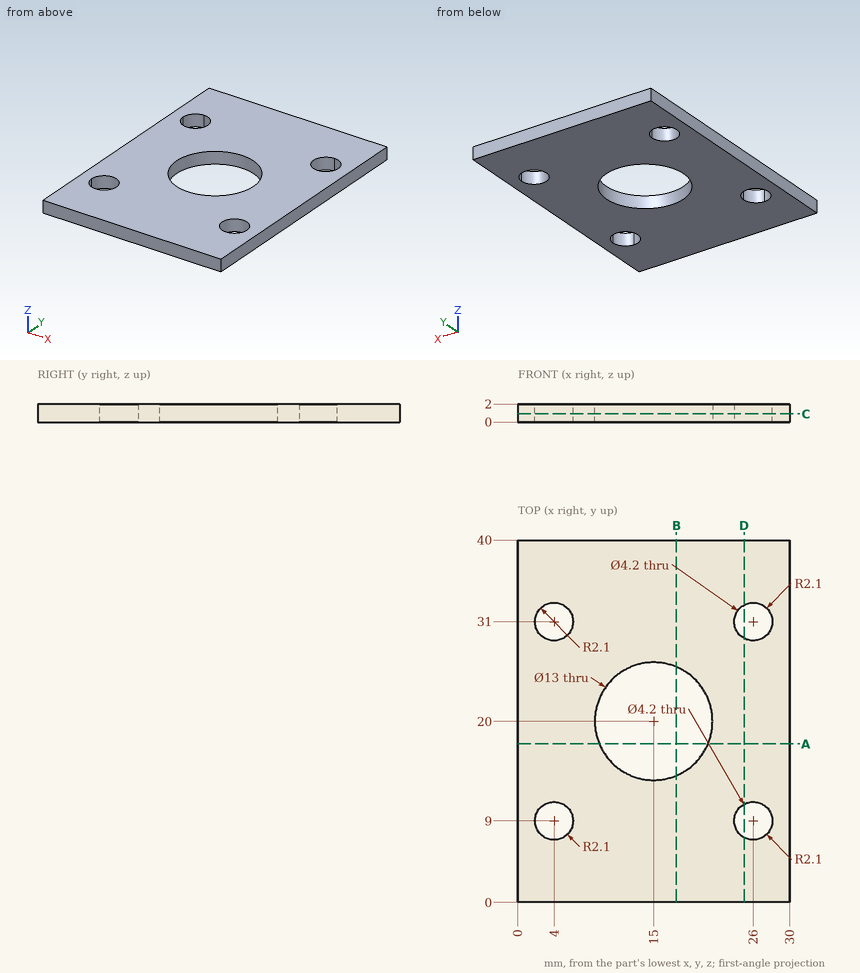
Geometry check sheet. Reference: drawing and pictorial views, mm from the part's lowest x, y, z. Give positions to 0.01 mm unless a question says otherwise; leave off trailing zeros. Order: outer loops, then holes, each group sorted by start corner. A loop starts at its lowest first (then second) coordinate and runs counter-clockwise, first axis right, second up. Notation, with made-up numbers: M 68,77 L 104,77 A21 ccw 104,110 Z; hole C -9.5,28 d4. An arc over 180 degrees is marked long. Answer in a Markdown table with one row per item. Add a question column.
Item 1: Gauge pin test, flat end, axial feed: pin 1 (2.5 mm diameter, centred on x = 26, y = 31, fed in from +Z). Record the tip position at first contact, or that the pin passes through.
Item 2: Scan lines: probe 1 along X at (y, z) = (9, 0.75); probe 2 along Y at (x, z) = (26, 0.1); probe 3 along X at (y, z) = (30.5, 0.2). Record each from-to range of solid material in increasing order. Write a range as from..to.
Item 3: Section check A-A, the plane y = 17.5. Enter the section's corners in (x, z).
Item 4: Section check B-B, the plane x = 17.5. Enter the section's corners in (y, z), and give its area (3 significant figures).
Item 5: Section check D-D, the plane x = 25. Enter the section's corners in (y, z).
Item 6: Section check C-C, the plane z = 0.9. Enter the section's corners in (x, y), and give its area (3 significant figures).
Filled sheet:
| question | item | result |
|---|---|---|
| 1 | pin 1 | passes through |
| 2 | probe 1 | x = 0..1.9, 6.1..23.9, 28.1..30 |
| 2 | probe 2 | y = 0..6.9, 11.1..28.9, 33.1..40 |
| 2 | probe 3 | x = 0..1.96, 6.04..23.96, 28.04..30 |
| 3 | outline | M 0,0 L 9,0 L 9,2 L 0,2 Z; M 21,0 L 30,0 L 30,2 L 21,2 Z |
| 4 | outline | M 0,0 L 14,0 L 14,2 L 0,2 Z; M 26,0 L 40,0 L 40,2 L 26,2 Z |
| 4 | area | 56.0 mm^2 |
| 5 | outline | M 0,0 L 7.15,0 L 7.15,2 L 0,2 Z; M 10.85,0 L 29.15,0 L 29.15,2 L 10.85,2 Z; M 32.85,0 L 40,0 L 40,2 L 32.85,2 Z |
| 6 | outline | M 0,0 L 30,0 L 30,40 L 0,40 Z; hole C 4,9 d4.2; hole C 4,31 d4.2; hole C 15,20 d13; hole C 26,9 d4.2; hole C 26,31 d4.2 |
| 6 | area | 1,010 mm^2 |
